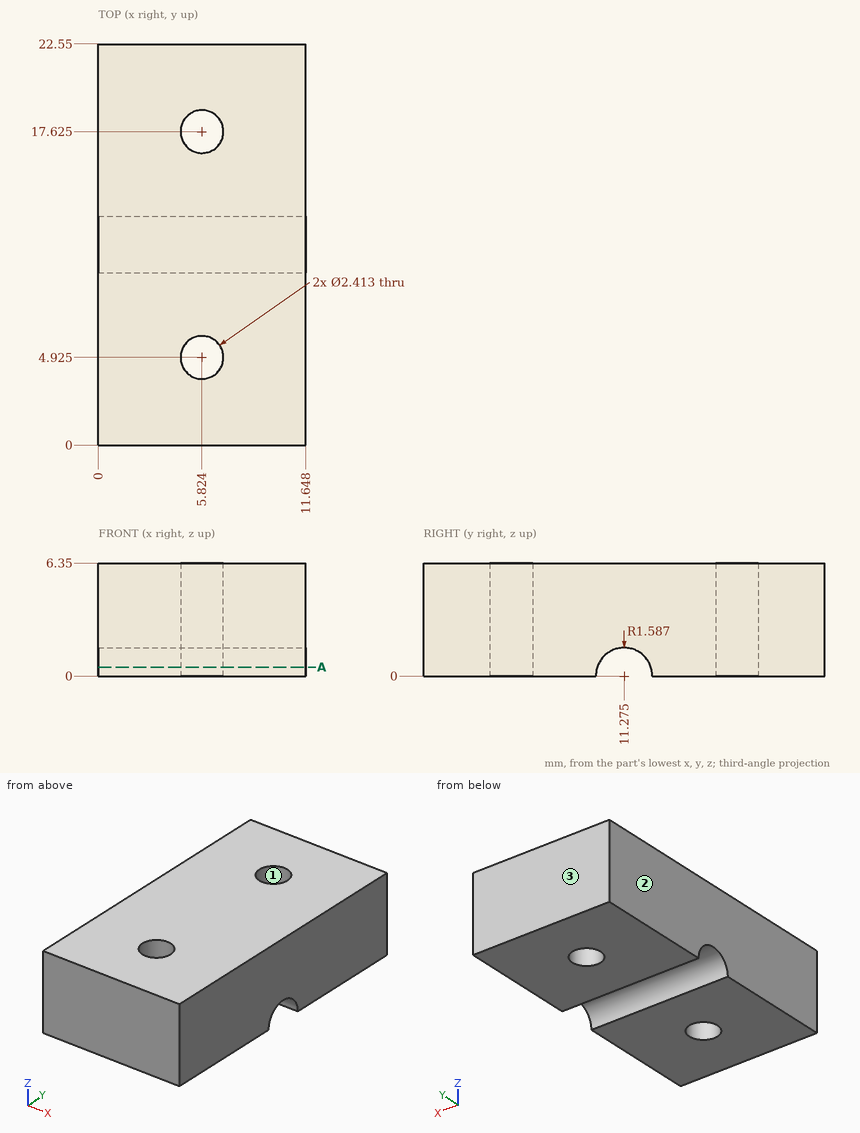
Job drawing, mm, ordinate dimensions from the low corner. One solid piece. Give positions to 0.01 mm unless a question says otherwise; leave off trailing zeros.
Item 1: Flat gauge pin, fed straight in: pin 1 (1.9 mm diameter, centred on x = 5.82, y = 17.62, fed in from +Z) (3 decimals). Where does the tip first touch, or does it go through?
Answers follow:
pin 1: passes through
Item 2: Slice it at A-A, the plane z = 0.5. Give the number of separate pieces and of enclosed holes in the cut face.
Answers follow:
separate pieces: 2
enclosed holes: 2
Item 3: Drill centre lines: line 1 (Y direction, x = 5.5, z = 5.5); line 2 (X direction, y = 5.25, z = 4.25) (1 decimal); line 3 (X direction, y = 17.5, z = 2) (1 decimal). Where is each one in solid material? Low to high.
Answers follow:
line 1: y = 0 to 3.76, 6.09 to 16.46, 18.79 to 22.55
line 2: x = 0 to 4.7, 7 to 11.6
line 3: x = 0 to 4.6, 7 to 11.6
Item 4: Pull direction X, two halves, no side cores. Call the marked faces 1, 2 and 3: released by +X, released by -X, zero draft, split by the parting line, or undercut.
Answers follow:
face 1: undercut
face 2: released by -X
face 3: zero draft
